Drawing for the job (mm, zero at the part's lowest x, y, z). A direction names the side the tool comes from. Give positions to 0.01 mm unless a question says otherwise; leave off trailing zeros. Order: outer loops, then holes, each group sorted by start corner. A loop starts at its lowest first (then second) coordinate and runs counter-clockwise, first axis right, second up. Notation, with made-up numbers: (84.25, -6.5) - (111.25, -6.5) arc R30 ccw to (111.25, 22.5) - close; hole circle Ø10 at (-27.5, 87). An arc over 180 degrees is marked (long way). One line per item, written item: value.
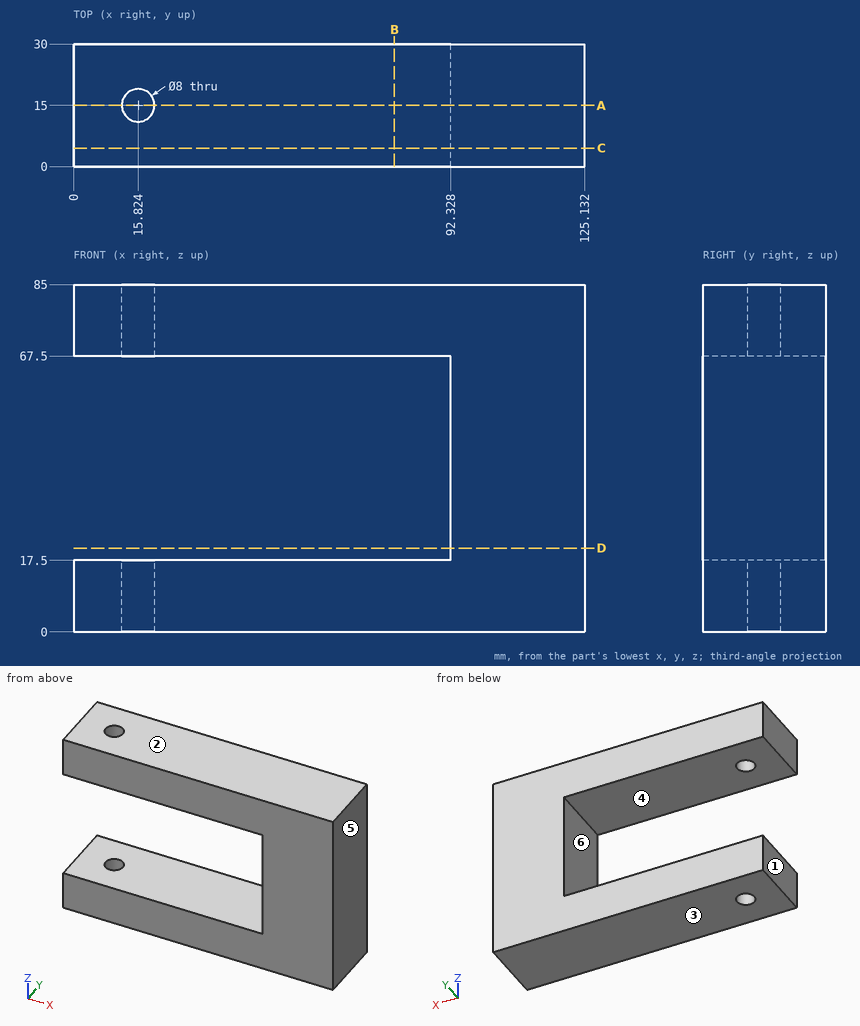
1) Cut at D-D, the plane z = 20.5. Give the cut face in (x, y).
Outcome:
outline: (92.33, 0) - (125.13, 0) - (125.13, 30) - (92.33, 30) - close
2) Which spindle directions (+Z, -Z, +X, -X, +Y, -Y) get a long thin tool onto all of the face, cutting with end or side? Do the marked faces 5 and 6. Say none if no direction does.
Outcome:
face 5: +Z, -Z, +X, +Y, -Y
face 6: -X, +Y, -Y
3) Drill centre lines: line 1 along Z through (x, y) = (91, 24.5); line 2 along X through (y, z) = (17.5, 47.5). Where is each one in solid material? Low to high. Write a range as from..to.
Outcome:
line 1: z = 0..17.5, 67.5..85
line 2: x = 92.33..125.13
4) Cut at C-C, the plane y = 4.5. Give the cut face in (x, z), then the cut area to 3 significant figures.
Outcome:
outline: (0, 0) - (125.13, 0) - (125.13, 85) - (0, 85) - (0, 67.5) - (92.33, 67.5) - (92.33, 17.5) - (0, 17.5) - close
area: 6,020 mm^2
5) Mould opens along Z. For the marked faces 1, 2, 3 and 4 say: released by +Z, released by -Z, zero draft, split by the parting line, or undercut.
Outcome:
face 1: zero draft
face 2: released by +Z
face 3: released by -Z
face 4: undercut
6) Cut at B-B, the plane x = 78.5. Give the cut face in (y, z), then the cut area to 3 significant figures.
Outcome:
outline: (0, 0) - (30, 0) - (30, 17.5) - (0, 17.5) - close; (0, 67.5) - (30, 67.5) - (30, 85) - (0, 85) - close
area: 1,050 mm^2
7) Cut at A-A, the plane y = 15. Give the cut face in (x, z).
Outcome:
outline: (0, 0) - (11.82, 0) - (11.82, 17.5) - (0, 17.5) - close; (0, 67.5) - (11.82, 67.5) - (11.82, 85) - (0, 85) - close; (19.82, 0) - (125.13, 0) - (125.13, 85) - (19.82, 85) - (19.82, 67.5) - (92.33, 67.5) - (92.33, 17.5) - (19.82, 17.5) - close
8) Pin check, flat tip, straight feed: pin 1 (1 mm diameter, centred on y = 11, z = 44, fed in from -X). Stop position of the tip, or through.
Outcome:
pin 1: stops at x = 92.33
